```python
from build123d import *

# Parameters (mm, degrees)
DIN_RAIL_NS_35_7_5_PERF_2000MM_1_DEPTH = 123.75


with BuildPart() as part:
    # Sketch12 → Din_rail NS 35 7 5 PERF 2000MM(1) (new body)
    with BuildSketch(Plane(origin=(0, 0, 0), x_dir=(-1, 0, 0), z_dir=(0, 0, -1))):
        with BuildLine():
            Line((11.7, 0), (-11.7, 0))
            ThreePointArc((-11.7, 0), (-12.972792206, 0.527207794), (-13.5, 1.8))
            Line((-13.5, 1.8), (-13.5, 5.7))
            ThreePointArc((-13.5, 5.7), (-13.734314575, 6.265685425), (-14.3, 6.5))
            Line((-14.3, 6.5), (-17.5, 6.5))
            Line((-17.5, 6.5), (-17.5, 7.5))
            Line((-17.5, 7.5), (-14.3, 7.5))
            ThreePointArc((-14.3, 7.5), (-13.027207794, 6.972792206), (-12.5, 5.7))
            Line((-12.5, 5.7), (-12.5, 1.8))
            ThreePointArc((-12.5, 1.8), (-12.265685425, 1.234314575), (-11.7, 1))
            Line((-11.7, 1), (11.7, 1))
            ThreePointArc((11.7, 1), (12.265685425, 1.234314575), (12.5, 1.8))
            Line((12.5, 1.8), (12.5, 5.7))
            ThreePointArc((12.5, 5.7), (13.027207794, 6.972792206), (14.3, 7.5))
            Line((14.3, 7.5), (17.5, 7.5))
            Line((17.5, 7.5), (17.5, 6.5))
            Line((17.5, 6.5), (14.3, 6.5))
            ThreePointArc((14.3, 6.5), (13.734314575, 6.265685425), (13.5, 5.7))
            Line((13.5, 5.7), (13.5, 1.8))
            ThreePointArc((13.5, 1.8), (12.972792206, 0.527207794), (11.7, 0))
        make_face()
    extrude(amount=DIN_RAIL_NS_35_7_5_PERF_2000MM_1_DEPTH)


solid = part.part
```
Design review of the part built by this model. Coordinates are the model's own, in mm. A direction names the side the tool comes from. Give positions to 0.01 mm unless a question says otherwise; leave off trailing zeros. Write each loop counter-clockwise with the first axis right and the second up, starting at its lowest first coordinate (ties: lowest second). Pieces come first, ordered by that corner, then holes. Notation, with made-up numbers: (74.25, -33) - (126.25, -33) arc R23 ccw to (126.25, -18) - close; hole circle Ø11 at (-25.75, 62). An arc over 180 degrees is marked (long way). Return JSON: item names as keys, results as strings. Group by question number.
(1) Insertion check: pin 1 (18.5 mm diameter, centred on x = -1, z = -61, fed in from +Y); pin 2 (3.5 mm diameter, centred on x = 16.5, z = -40, fed in from -Y); pin 3 (1.5 mm diameter, centred on y = 1, z = -59, fed in from -X); pin 4 (1 mm diameter, centred on x = -6.5, y = 2.5, fed in from +Z). Each pin has a flat end and moves straight along its axis. Give the tip position at first contact, or say it passes through.
(2) Machinability: for faces 1 (the flat face through (-12.5, 4, -61)), 2 (the flat face through (0, 0, -61)), 3 (the flat face through (13.5, 4, -61)), which of the approach directions +Z, -Z, +X, -X, +Y, -Y give a long, thin tool a straight path to every point of the face, cutting with its end or side? Answer none if there is none.
(3) To check wall thickness, follow probe 1 along X at (y, z) = (4, -35.5); probe 2 along Y at (x, z) = (-9, -101); probe 3 along X at (y, z) = (7.25, -75.5). State the ranges of each line that lie inside material, in increasing order.
(4) Mouldability with a two-part tool opening along X and no side actions: class faces 4 (the flat face through (12.5, 4, -61)), 5 (the flat face through (-16, 6.5, -61)), 6 (the flat face through (0, 1, -61)), 7 (the flat face through (-13.5, 4, -61)) as +X half, -X half, draft (parallel to the pull), parting line (faces both ways), or undercut.
(5) We need section B-B, the plane x = 1.5. Give the boundary of the cut face in (y, z), then the cut area to 3 significant figures.
(6) We need section A-A, the plane z = -36. Give the boundary of the cut face in (x, y).
Reported:
{
 "1": {"pin 1": "stops at y = 1", "pin 2": "stops at y = 6.5", "pin 3": "stops at x = -13.5", "pin 4": "passes through"},
 "2": {"face 1": "+Z, -Z, +Y", "face 2": "+Z, -Z, +X, -X, -Y", "face 3": "+Z, -Z, +X, -Y"},
 "3": {"probe 1": "x = -13.5 to -12.5, 12.5 to 13.5", "probe 2": "y = 0 to 1", "probe 3": "x = -17.5 to -13.38, 13.38 to 17.5"},
 "4": {"face 4": "undercut", "face 5": "draft", "face 6": "undercut", "face 7": "-X half"},
 "5": {"outline": "(0, -123.75) - (1, -123.75) - (1, 0) - (0, 0) - close", "area": "124 mm2"},
 "6": {"outline": "(-17.5, 6.5) - (-14.3, 6.5) arc R0.8 cw to (-13.5, 5.7) - (-13.5, 1.8) arc R1.8 ccw to (-11.7, 0) - (11.7, 0) arc R1.8 ccw to (13.5, 1.8) - (13.5, 5.7) arc R0.8 cw to (14.3, 6.5) - (17.5, 6.5) - (17.5, 7.5) - (14.3, 7.5) arc R1.8 ccw to (12.5, 5.7) - (12.5, 1.8) arc R0.8 cw to (11.7, 1) - (-11.7, 1) arc R0.8 cw to (-12.5, 1.8) - (-12.5, 5.7) arc R1.8 ccw to (-14.3, 7.5) - (-17.5, 7.5) - close"}
}
